Verification items for the finished model (mm, model axes). A direction names the side the tool comes from. Coordinates: 2 decimals unless noted, no trailing zeros. Write each loop counter-clockwise with the first axis right and the second up, starting at its lowest first coordinate (ties: lowest second). Pieces come first, ordered by that corner, then holes. Notation, with made-up numbers: M 3.25,69 L 41.25,69 A30 cw 41.25,102 Z; hole C -9.75,16.25 d1. An arc over 180 degrees is marked long. Answer in a Markdown table with one row per item.
Autodesk Inventor part; units mm, degrees
ref_plane "Work Plane2" through (3.35, 0, 0) normal (0, 0, -1) x (1, 0, 0)
ref_plane "YZ Plane" through (0, 0, 0) normal (1, 0, 0) x (0, 1, 0)
ref_plane "XZ Plane" through (0, 0, 0) normal (0, 1, 0) x (-1, 0, 0)
sketch "Sketch1" plane through (0, 0, 0) normal (0, 0, 1) x (1, 0, 0)
  line L0 (2.1, 0) -> (14, 0)
  line L1 (14, 0) -> (14, 1.5)
  line L2 (14, 1.5) -> (2.65, 1.5)
  line L3 (2.65, 1.5) -> (2.3433, 1.3466)
  line L4 (2.3433, 1.3466) -> (1.9814, 1.3466)
  line L5 (0, 2.75) -> (0, 1.6)
  line L6 (0, 1.6) -> (1.6999, 0.7525)
  line L7 (1.6999, 0.7525) -> (2.1, 0)
  line L8 (-2.8, 0) -> (16.8, 0)
  line L9 (0, -0.55) -> (0, 3.3)
  line L10 (0, 2.75) -> (0.2466, 2.75)
  line L11 (0.2466, 2.75) -> (1.4157, 1.581)
  line L12 (2.65, 1.5) -> (1.4966, 1.5) construction
  arc A0 (1.4157, 1.581) -> (1.9814, 1.3466) centre (1.9814, 2.1466) ccw
  point P0 (1.65, 1.3466)
  dimension "d1" = 11.35
  dimension "d2" = 3
  dimension "d3" = 2.6933
  dimension "d4" = 3.2
  dimension "d5" = 26.5
  dimension "d6" = 62
  dimension "d7" = 2.1
  dimension "d8" = 0.3067
  dimension "d12" = 5.5
  dimension "d13" = 45
  dimension "d15" = 14
  dimension "d24" = 1.65
  dimension "d93" = 0.8
revolve "Body" add sketch "Sketch1" angle 360 about axis through (2.1, 0, 0) along (1, 0, 0) contours L7 L6 L5 L10 L11 A0 L4 L3 L2 L1 L0
sketch "Sketch2" plane through (0, 0, 0) normal (-1, 0, 0) x (0, 0, 1)
  line L0 (0, 1.6) -> (0, 0) construction
  line L1 (0, 0) -> (1.6, 0) construction
  arc A0 (0.48, 0) -> (0, 0.48) centre (0, 0) ccw construction
  arc A1 (0.56, 0) -> (0, 0.56) centre (0, 0) ccw construction
  arc A2 (1.5795, 0.255) -> (0.255, 1.5795) centre (0, 0) ccw
  line L2 (0, 0) -> (1.1314, 1.1314) construction
  line L3 (0.255, 1.5795) -> (0.2766, 0.4869)
  line L4 (1.5795, 0.255) -> (0.4869, 0.2766)
  arc A3 (0.255, 1.5795) -> (0, 1.6) centre (0, 0) ccw
  arc A4 (1.6, 0) -> (1.5795, 0.255) centre (0, 0) ccw
  line L5 (0, -3.85) -> (0, 3.85)
  line L6 (-3.85, 0) -> (3.85, 0)
  arc A5 (0.255, -1.5795) -> (1.5795, -0.255) centre (0, 0) ccw
  line L7 (0.255, -1.5795) -> (0.2766, -0.4869)
  line L8 (1.5795, -0.255) -> (0.4869, -0.2766)
  arc A6 (0, -1.6) -> (0.255, -1.5795) centre (0, 0) ccw
  arc A7 (1.5795, -0.255) -> (1.6, 0) centre (0, 0) ccw
  arc A8 (-0.255, 1.5795) -> (-1.5795, 0.255) centre (0, 0) ccw
  line L9 (-0.255, 1.5795) -> (-0.2766, 0.4869)
  line L10 (-1.5795, 0.255) -> (-0.4869, 0.2766)
  arc A9 (0, 1.6) -> (-0.255, 1.5795) centre (0, 0) ccw
  arc A10 (-1.5795, 0.255) -> (-1.6, 0) centre (0, 0) ccw
  arc A11 (-0.255, -1.5795) -> (0, -1.6) centre (0, 0) ccw
  arc A12 (-1.5795, -0.255) -> (-0.255, -1.5795) centre (0, 0) ccw
  arc A13 (-1.6, 0) -> (-1.5795, -0.255) centre (0, 0) ccw
  line L11 (-1.5795, -0.255) -> (-0.4869, -0.2766)
  line L12 (-0.255, -1.5795) -> (-0.2766, -0.4869)
  arc A14 (0.2766, 0.4869) -> (0.4869, 0.2766) centre (0.4912, 0.4912) ccw
  arc A15 (0.4869, -0.2766) -> (0.2766, -0.4869) centre (0.4912, -0.4912) ccw
  arc A16 (-0.4869, 0.2766) -> (-0.2766, 0.4869) centre (-0.4912, 0.4912) ccw
  arc A17 (-0.2766, -0.4869) -> (-0.4869, -0.2766) centre (-0.4912, -0.4912) ccw
  point P0 (1.1314, -1.1314)
  point P1 (-1.1314, 1.1314)
  point P2 (-1.1314, -1.1314)
  dimension "d17" = 0.96
  dimension "d18" = 1.12
  dimension "d19" = 3.2
  dimension "d20" = 45
  dimension "d21" = 0.255
extrude "Slot" add sketch "Sketch2" against normal up to next draft 5 contours L4 A14 L3 A2 | A5 L7 A15 L8 | L9 A16 L10 A8 | A12 L11 A17 L12
fillet "Fillet1" radius 0.102 4 edges at (0, 1.6, 0) (0, 0, -1.6) (0, -1.6, 0) (0, 0, 1.6)
thread "Thread"
chamfer "Chamfer1" distance 0.3067 distance2 0.1534 1 edges at (14, -1.5, 0) measured on face at (14, 0.263, 0.1197)
ref_plane "Work Plane2" through (3.35, 0, 0) normal (0, 0, -1) x (1, 0, 0)
equation "\"d1\" = GEL"
equation "\"d2\" = GD"
equation "\"d3\" = BDM"
equation "\"d4\" = SDM"
equation "\"d7\" = INTI"
equation "\"d8\" = GAL"
equation "\"d12\" = KOD"
equation "\"d13\" = 0.5 * SEWI"
equation "\"d15\" = NLG"
equation "\"d93\" = R"
equation "\"d17\" = 0.3 * SDM"
equation "\"d18\" = 0.35 * SDM"
equation "\"d19\" = SDM"
equation "\"d21\" = 0.5 * SBR"
equation "\"d23\" = 0.2 * SBR"
equation "\"d10\" = GEL"
equation "\"d25\" = -0.5 * SPD + 0.5 * GD"
equation "\"d26\" = 0.5 * GAL"
equation "\"NLG\" = 14"
equation "\"GEL\" = 11.35"
equation "\"GAL\" = 0.61345 * PTC"
equation "\"SPD\" = NND - 1.2269 * PTC"
equation "\"KOD\" = 5.5"
equation "\"KOH\" = 1.65"
equation "\"SBR\" = 0.51"
equation "\"INTI\" = 2.1"
equation "\"SDM\" = 3.2"
equation "\"GD\" = NND"
equation "\"BDM\" = NND - GAL"
equation "\"SEWI\" = 90deg"
equation "\"d9\" = SDM"
equation "\"R\" = 0.8"
equation "\"GUL\" = 0.61345 * PTC"
equation "\"TOA\" = 30deg"
equation "\"EPV\" = 3.15"
equation "\"THREADDIA\" = 3"
equation "\"PTC\" = 0.5"
equation "\"NND\" = 3"
equation "\"GD1\" = THREADDIA - 1.2269 * PTC"
properties part number "ISO 7046-1  - M3 x 14 - 4.8 - H" material "Steel"
1) Release check for a two-part mould opening along Y. For faces 1 (the face through (2.03, -0.1, -0.09)), 2 (the face through (14, 0, 0)), 3 (the face through (8.17, -1.5, -0.07)), 4 (the face through (0.867, -0.003, 1.168)) record: +Y half, -Y half, draft (parallel to the pull), parting line (faces both ways), or undercut.
Response values:
| item | result |
|---|---|
| face 1 | undercut |
| face 2 | draft |
| face 3 | parting line |
| face 4 | undercut |
2) Tool access check on faces 5 (the face through (2.16, -1.345, -0.059)), 6 (the face through (0, 1, -1)), 7 (the face through (0.867, 0.003, -1.168)). Record the directions out of +Z, -Z, +X, -X, +Y, -Y that give a thin tool (end or side, any length) a straight path to the whole face; none if there is none.
Response values:
| item | result |
|---|---|
| face 5 | none |
| face 6 | +Z, -Z, -X, +Y, -Y |
| face 7 | -X |
3) Thickness scan on L1, parallel to X at y = 0.75, z = 1.2; L2, parallel to Y at x = 1.25, z = 1.5; L3, parallel to X at y = 2.5, z = 0.85. Record the ranges inside material, lowest first. Write a range as [from, to].
Response values:
| item | result |
|---|---|
| L1 | x = [0, 1.66], [2.48, 13.89] |
| L2 | y = [-0.89, 0.89] |
| L3 | x = [0, 0.36] |
4) Sectioned sample at B-B (x = 4.5). Record the cut outline in (y, z), then the cut area to 3 significant figures.
Response values:
| item | result |
|---|---|
| outline | C 0,0 d3 |
| area | 7.07 mm² |
5) Sectioned sample at A-A (x = 1). Record the cut outline in (y, z), then the cut area to 3 significant figures.
Response values:
| item | result |
|---|---|
| outline | C 0,0 d3.99; hole M -1.09,-0.18 L -0.49,-0.19 A0.3 cw -0.19,-0.49 L -0.18,-1.09 A1.1 ccw 0.18,-1.09 L 0.19,-0.49 A0.3 cw 0.49,-0.19 L 1.09,-0.18 A1.1 ccw 1.09,0.18 L 0.49,0.19 A0.3 cw 0.19,0.49 L 0.18,1.09 A1.1 ccw -0.18,1.09 L -0.19,0.49 A0.3 cw -0.49,0.19 L -1.09,0.18 A1.1 ccw Z |
| area | 11.0 mm² |
